Verification items for the finished model (mm, model axes). Coordinates: 2 decimals unless noted, no trailing zeros. Loops run counter-clockwise (first coordinate to the right, second up) from the corner with the lowest first, then second, coordinate; pieces in that order, holes last.
Q1. Go/stop test with a flat-tipped pin: P1, Ø1.5, axis at x = -2, z = -3.5, coming from the -Y side. Record where the tip stops, or that it passes through.
Q2. Sectioned sample at D-D (x = -5.08). Enter the section's corners in (y, z).
Q3. Mould release check, pull along Z, two halves, no side actions. Record for faces 1 (the face through (8.126, 12.878, -5.308)), 2 (the face through (-8.706, 12.878, -1.493)), 3 (the face through (1.92, 12.52, 1.2)): +Z half, -Z half, draft (parallel to the pull), parting line (faces both ways), or undercut.
Q4. Sectioned sample at C-C (y = 13.75). Count the separate pieces of the cut face and the enclosed holes in it, then the cut area to 3 significant figures.
Q5. Sectioned sample at B-B (z = 2). Enter the section's corners in (x, y), then the cut area to 3 significant figures.
Q6. Sectioned sample at A-A (x = 3.81). Enter the section's corners in (y, z), then the cut area to 3 significant figures.
Q7. Material ranges on probe 1 along X at (y, z) = (2.5, 1.5); probe 2 along X at (y, z) = (14, 2.25); probe 3 along Z at (x, y) = (-6, 17), recorded low to high.
```python
from build123d import *

# Parameters (mm, degrees)
SKETCH1_W           = 17.78
SKETCH1_H           = 12.065
SKETCH1_R           = 1.905
BOSS_EXTRUDE1_DEPTH = 25.4
CUT_EXTRUDE1_DEPTH  = 28.578672126
FILLET1_R           = 2.54
FILLET2_R           = 12.7


with BuildPart() as part:
    # Sketch1 → Boss-Extrude1 (new body)
    with BuildSketch(Plane(origin=(0, 0, 0), x_dir=(1, 0, 0), z_dir=(0, 1, 0))):
        Rectangle(SKETCH1_W, SKETCH1_H)
        with Locations(Location((-5.08, -0.9525, 0), (0, 0, 270))):
            Circle(SKETCH1_R, mode=Mode.SUBTRACT)
        with Locations(Location((3.81, -0.9525, 0), (0, 0, 90))):
            Circle(SKETCH1_R, mode=Mode.SUBTRACT)
    extrude(amount=BOSS_EXTRUDE1_DEPTH)

    # Sketch2 → Cut-Extrude1 (cut, through all)
    with BuildSketch(Plane(origin=(0, 25.4, 0), x_dir=(1, 0, 0), z_dir=(0, 1, 0))):
        Polygon((-8.89, 1.5875), (-6.35, -6.0325), (-8.89, -6.0325), align=None)
    extrude(amount=-CUT_EXTRUDE1_DEPTH, mode=Mode.SUBTRACT)

    # Fillet1
    fillet1_edges = [part.edges().sort_by_distance(p)[0] for p in [
        (-6.35, 12.7, 6.0325),
        (8.89, 12.7, 6.0325),
        (-8.89, 12.7, -6.0325),
        (8.89, 12.7, -6.0325),
    ]]
    fillet(fillet1_edges, radius=FILLET1_R)

    # Fillet2
    # the kernel refuses this fillet: 12.7 mm, written as the material it takes off along each edge
    with BuildSketch(Plane(origin=(-8.89, 30.542393541, -1.5875), x_dir=(0.00016823247484796397, 0, -0.9999999858489171), z_dir=(0, -1, 0))) as fillet2_piece_1:
        with BuildLine():
            CenterArc((2.066827795, 12.698397406), FILLET2_R, 251.555412166, 17.534355835)
            Line((-1.951291688, 0.650795328), (-2.353103637, -0.553964879))
            Line((-2.353103637, -0.553964879), (-0.401811948, -1.204760208))
            Line((-0.401811948, -1.204760208), (-0.000213655, -1.269999982))
            ThreePointArc((-0.000213655, -1.269999982), (1.904786318, -1.270320465), (1.844902092, -1.269839741))
            Line((1.844902092, -1.269839741), (1.865077156, 0))
        make_face()
    extrude(amount=35.684787082, mode=Mode.SUBTRACT)


solid = part.part
```
Geometry check:
1. P1: stops at y = 0
2. outline: (0, -6.03) - (25.4, -6.03) - (25.4, -0.95) - (0, -0.95) - close; (0, 2.86) - (25.4, 2.86) - (25.4, 5.97) - (0, 5.97) - close
3. face 1: -Z half
3. face 2: +Z half
3. face 3: undercut
4. separate pieces: 1
4. enclosed holes: 2
4. area: 177 mm2
5. outline: (-7.69, 0) - (-6.67, 0) - (-6.67, 25.4) - (-7.69, 25.4) - close; (-3.49, 0) - (2.22, 0) - (2.22, 25.4) - (-3.49, 25.4) - close; (5.4, 0) - (8.89, 0) - (8.89, 25.4) - (5.4, 25.4) - close
5. area: 260 mm2
6. outline: (0, -6.03) - (25.4, -6.03) - (25.4, -0.95) - (0, -0.95) - close; (0, 2.86) - (25.4, 2.86) - (25.4, 6.03) - (0, 6.03) - close
6. area: 210 mm2
7. probe 1: x = -7.86 to -6.9, -3.26 to 1.99, 5.63 to 8.89
7. probe 2: x = -7.61 to -6.47, -3.69 to 2.42, 5.2 to 8.89
7. probe 3: z = -6.03 to -0.72, 2.62 to 5.56
